from build123d import *

# Parameters (mm, degrees)
F0_W      = 20
F0_H      = 20
F1_DEPTH  = 20
F2_R      = 6.297785
F3_DEPTH  = 16.5
F4_R      = 5.5
F5_DEPTH  = 16.5
F6_R      = 3.57
F7_DEPTH  = 20.001
F8_R      = 3.57
F9_DEPTH  = 20.001
F11_DEPTH = 20.001


with BuildPart() as f1:
    # F0 (on Top) → F1 (new body)
    with BuildSketch(Plane.XY):
        Rectangle(F0_W, F0_H)
    extrude(amount=F1_DEPTH)

    # F2 (on face) → F3 (cut)
    with BuildSketch(Plane.YZ.offset(10)):
        with Locations((0, 10)):
            Circle(F2_R)
    extrude(amount=-F3_DEPTH, mode=Mode.SUBTRACT)

    # F4 (on face) → F5 (cut)
    with BuildSketch(Plane.XY.offset(20)):
        Circle(F4_R)
    extrude(amount=-F5_DEPTH, mode=Mode.SUBTRACT)

    # F6 (on face) → F7 (cut, through all)
    with BuildSketch(Plane(origin=(0, 0, 0), x_dir=(1, 0, 0), z_dir=(0, 0, -1))):
        Circle(F6_R)
    extrude(amount=-F7_DEPTH, mode=Mode.SUBTRACT)

    # F8 (on face) → F9 (cut, through all)
    with BuildSketch(Plane(origin=(-10, 0, 0), x_dir=(0, -1, 0), z_dir=(-1, 0, 0))):
        with Locations((0, 10)):
            Circle(F8_R)
    extrude(amount=-F9_DEPTH, mode=Mode.SUBTRACT)

    # F10 (on face) → F11 (cut, through all)
    with BuildSketch(Plane(origin=(0, 10, 0), x_dir=(-1, 0, 0), z_dir=(0, 1, 0))):
        Polygon((9, 20), (-10, 20), (-10, 1), align=None)
    extrude(amount=-F11_DEPTH, mode=Mode.SUBTRACT)


solid = f1.part
Here's how the part is built. I have some questions about the finished solid (model axes, mm). A direction names the side the tool comes from. Coordinates: 2 decimals unless noted, no trailing zeros. Order: outer loops, then holes, each group sorted by start corner. A loop starts at its lowest first (then second) coordinate and runs counter-clockwise, first axis right, second up. Notation, with made-up numbers: (86.25, -23.75) - (139.25, -23.75) arc R12 cw to (139.25, -15.75) - close; hole circle Ø2 at (-20, -10). An arc over 180 degrees is marked (long way). Use CSV: the item, a comma, the result in double quotes. Start each with the question number.
1. Suppose I cut it at A-A on z = 10. List the corners of the cut face in (x, y) for me.
2. Suppose I cut it at D-D on z = 3. List the corners of the cut face in (x, y) for me, then the cut area to 3 significant figures.
3. Suppose I cut it at C-C on x = 2.75. List the corners of the cut face in (y, z) for me.
4. Suppose I cut it at B-B on y = 0. List the corners of the cut face in (x, z) for me.
5. For faces 1 (the face through (-2.64, 5.21, 6.46)), 2 (the face through (-0.716, 5.453, 4.859)), 3 (the face through (-9.5, 0.1, 20)), which set-ups out of +Z, -Z, +X, -X, +Y, -Y let a thin tool reach every point of the face, with its end or its side?
6. I'm going to push flat-ended pins straight in: pin 1 (8 mm diameter, centred on y = 0, z = 10, fed in from +X); pin 2 (11.5 mm diameter, centred on x = 0, y = 0, fed in from +Z); pin 3 (12 mm diameter, centred on y = 6, z = 16.5, fed in from +X); pin 4 (3.5 mm diameter, centred on x = -0.5, y = -1, fed in from +Z) (1 decimal). Where does each tip first touch, or does it pass through?
7. If we mould it in two halves opening along X, with no side actions, what happens to faces 4 (the face through (4, 0, 3.5)), 5 (the face through (-2, 10, 8)), 6 (the face through (-6.5, 3, 7))? For each: +X half, -X half, draft (parallel to the pull), parting line (faces both ways), or undercut.
8. Please list where these lines run through material, in increasing order: line 1 (Y direction, x = 0, z = 1.5); line 2 (Y direction, x = -0.25, z = 10); line 3 (X direction, y = -1, z = 17.5). Write a range as from..to.
Output:
1,outline,"(-10, -10) - (1, -10) - (1, -6.3) - (-6.5, -6.3) - (-6.5, -3.57) - (-10, -3.57) - close; (-10, 3.57) - (-6.5, 3.57) - (-6.5, 6.3) - (1, 6.3) - (1, 10) - (-10, 10) - close"
2,outline,"(-10, -10) - (8, -10) - (8, 10) - (-10, 10) - close; hole circle Ø7.14 at (0, 0)"
2,area,"320 mm2"
3,outline,"(-10, 0) - (-2.28, 0) - (-2.28, 3.5) - (-4.76, 3.5) - (-4.76, 5.88) arc R6.3 cw to (-6.05, 8.25) - (-10, 8.25) - close; (2.28, 0) - (10, 0) - (10, 8.25) - (6.05, 8.25) arc R6.3 cw to (4.76, 5.88) - (4.76, 3.5) - (2.28, 3.5) - close"
4,outline,"(-10, 0) - (-3.57, 0) - (-3.57, 3.5) - (-5.5, 3.5) - (-5.5, 3.7) - (-6.5, 3.7) - (-6.5, 6.43) - (-10, 6.43) - close; (-10, 13.57) - (-6.5, 13.57) - (-6.5, 16.3) - (-5.5, 16.3) - (-5.5, 16.5) - (-9, 20) - (-10, 20) - close; (3.57, 0) - (10, 0) - (10, 1) - (7.3, 3.7) - (5.5, 3.7) - (5.5, 3.5) - (3.57, 3.5) - close"
5,face 1,"+X"
5,face 2,"+Z"
5,face 3,"+Z, +X, -X, +Y, -Y"
6,pin 1,"stops at x = -6.5"
6,pin 2,"stops at z = 16.75"
6,pin 3,"stops at x = 0.49"
6,pin 4,"passes through"
7,face 4,"undercut"
7,face 5,"draft"
7,face 6,"+X half"
8,line 1,"y = -10..-3.57, 3.57..10"
8,line 2,"y = -10..-6.3, 6.3..10"
8,line 3,"x = -10..-6.5"
